Autodesk Inventor part; units mm, degrees
ref_plane "Work Plane1" through (34.6017, 22.9, 27.7) normal (0, 0, 1) x (0, -1, 0)
ref_plane "Work Plane3" through (19.1, 22.9, 27.7) normal (0, -1, 0) x (1, 0, 0)
ref_plane "Work Plane4" through (53.9, 4.4, -9.45) normal (1, 0, 0) x (0, 1, 0)
ref_plane "Work Plane1" through (34.6017, 22.9, 27.7) normal (0, 0, 1) x (0, -1, 0)
sketch "Sketch1" plane through (34.6017, 22.9, 27.7) normal (0, 0, 1) x (0, -1, 0)
  line L0 (-22.65, -5.5017) -> (22.65, -5.5017)
  line L1 (22.65, -5.5017) -> (22.65, -15.5017)
  line L2 (22.65, -15.5017) -> (-22.65, -15.5017)
  line L3 (-22.65, -15.5017) -> (-22.65, -5.5017)
  line L4 (-23.05, -33.7017) -> (-23.05, 15.1916) construction
  line L5 (23.05, 15.1916) -> (23.05, -33.7017) construction
  line L6 (-23.95, -33.6017) -> (-23.95, 15.3983) construction
  line L7 (22.9493, -34.6017) -> (-22.9493, -34.6017) construction
  line L8 (-23.85, -35.5017) -> (23.85, -35.5017) construction
  line L9 (23.05, -33.7017) -> (-23.05, -33.7017) construction
  point P0 (22.9, -34.6017)
  dimension "d0" = 45.3
  dimension "d1" = 10
  dimension "d2" = 0.4
  dimension "d4" = 20
extrude "Extrusion1" add sketch "Sketch1" along normal blind 3
sketch "Sketch2" plane through (19.1, 45.55, 27.7) normal (0, 1, 0) x (1, 0, 0)
  line L0 (10, 0) -> (10, -3)
  line L1 (0, -3) -> (10, -3)
  line L2 (10, -3) -> (10, -0.9)
  line L3 (10, -0.9) -> (0, -0.9)
  line L4 (0, -0.9) -> (0, -3)
  point P0 (-19.1, 27.7)
  dimension "d7" = 2.1
extrude "Extrusion2" add sketch "Sketch2" along normal blind 2
ref_plane "Work Plane3" through (19.1, 22.9, 27.7) normal (0, -1, 0) x (1, 0, 0)
mirror "Mirror2" about plane through (19.1, 22.9, 27.7) normal (0, -1, 0) of "Extrusion2"
sketch "Sketch3" plane through (19.1, 0.25, 27.7) normal (0, -1, 0) x (1, 0, 0)
  line L0 (10, 0.9) -> (0, 0.9)
  line L1 (0, 0) -> (0, 0.9)
  line L2 (10, 0) -> (0, 0)
  line L3 (10, 0) -> (10, 0.9)
  point P0 (-19.1, -27.7)
extrude "Extrusion3" add sketch "Sketch3" along normal blind 0.2
sketch "Sketch4" plane through (19.1, 45.55, 27.7) normal (0, 1, 0) x (1, 0, 0)
  line L0 (0, -0.9) -> (10, -0.9)
  line L1 (10, 0) -> (10, -0.9)
  line L2 (0, 0) -> (10, 0)
  line L3 (0, 0) -> (0, -0.9)
  point P0 (-19.1, 27.7)
extrude "Extrusion4" add sketch "Sketch4" along normal blind 0.2
sketch "Sketch5" plane through (19.1, 47.55, 27.7) normal (0, 1, 0) x (1, 0, 0)
  line L0 (0, -3) -> (10, -3)
  line L1 (10, -3) -> (10, -0.9)
  line L2 (10, -0.9) -> (0, -0.9)
  line L3 (0, -0.9) -> (0, -3)
  point P0 (-19.1, 27.7)
extrude "Extrusion5" add sketch "Sketch5" along normal blind 1.6
sketch "Sketch6" plane through (19.1, -1.75, 30.7) normal (0, -1, 0) x (1, 0, 0)
  line L0 (0, 0) -> (10, 0)
  line L1 (0, -2.1) -> (0, 0)
  line L2 (10, -2.1) -> (0, -2.1)
  line L3 (10, 0) -> (10, -2.1)
  point P0 (-19.1, -30.7)
extrude "Extrusion6" add sketch "Sketch6" along normal blind 1.6
sketch "Sketch7" plane through (29.1, 45.75, 28.6) normal (0, 0, -1) x (-1, 0, 0)
  line L0 (10, 0) -> (10, 3.4)
  line L1 (0, 3.4) -> (10, 3.4)
  line L2 (10, 3.4) -> (10, 1.85)
  line L3 (10, 1.85) -> (0, 1.85)
  line L4 (0, 1.85) -> (0, 3.4)
  point P0 (29.1, -45.75)
  dimension "d20" = 1.55
extrude "Extrusion7" add sketch "Sketch7" along normal up to surface (0.9 mm away)
mirror "Mirror3" about plane through (19.1, 22.9, 27.7) normal (0, -1, 0) of "Extrusion7"
sketch "Sketch8" plane through (19.1, 47.6, 28.6) normal (0, -1, 0) x (1, 0, 0)
  line L0 (0, -0.9) -> (10, -0.9)
  line L1 (10, 0) -> (10, -0.9)
  line L2 (0, 0) -> (10, 0)
  line L3 (0, 0) -> (0, -0.9)
  point P0 (-19.1, -28.6)
extrude "Extrusion8" cut sketch "Sketch8" against normal blind 0.2
sketch "Sketch9" plane through (19.1, -1.8, 27.7) normal (0, 1, 0) x (1, 0, 0)
  line L0 (0, 0) -> (10, 0)
  line L1 (0, -0.9) -> (0, 0)
  line L2 (10, -0.9) -> (0, -0.9)
  line L3 (10, -0.9) -> (10, 0)
  point P0 (-19.1, 27.7)
extrude "Extrusion9" cut sketch "Sketch9" against normal blind 0.2
sketch "Sketch10" plane through (34.6017, 22.9, 30.7) normal (0, 0, 1) x (1, 0, 0)
  line L0 (-5.5017, 26.25) -> (-5.5017, -26.25)
  line L1 (-15.5017, 26.25) -> (-5.5017, 26.25)
  line L2 (-15.5017, -26.25) -> (-15.5017, 26.25)
  line L3 (-5.5017, -26.25) -> (-15.5017, -26.25)
  point P0 (-34.6017, -22.9)
extrude "Extrusion10" add sketch "Sketch10" along normal blind 2
sketch "Sketch11" plane through (29.1, 0.05, 27.7) normal (1, 0, 0) x (0, 0, -1)
  line L0 (0, 45.7) -> (0, 0)
  line L1 (-5, -3.4) -> (-5, 49.1)
  line L2 (-5, 27.85) -> (0, 27.85)
  line L3 (0, 27.85) -> (0, 17.85)
  line L4 (0, 17.85) -> (-5, 17.85)
  line L5 (-5, 17.85) -> (-5, 27.85)
  line L6 (0, 49.1) -> (-5, 49.1)
  point P0 (27.7, -0.05)
  dimension "d29" = 10
  dimension "d37" = 21.25
ref_plane "Work Plane4" through (53.9, 4.4, -9.45) normal (1, 0, 0) x (0, 1, 0)
ref_plane "Work Plane5" through (56.9, 17.9, 20.2) normal (1, 0, 0) x (0, 1, 0)
extrude "Extrusion11" add sketch "Sketch11" along normal up to surface (27.8 mm away)
sketch "Sketch12" plane through (29.1, 17.9, 27.7) normal (0, -1, 0) x (1, 0, 0)
  line L0 (16.8, 0) -> (16.8, 0.8) construction
  line L1 (15.8, 0.8) -> (16.8, 0.8) construction
  line L2 (15, 0) -> (15, 0.8) construction
  line L3 (27.8, 0) -> (27.8, 5) construction
  line L4 (0, 5) -> (27.8, 5) construction
  line L5 (0, 0) -> (0, 5) construction
  line L6 (0, 0) -> (27.8, 0) construction
  line L7 (-34.3067, 0.8) -> (15.8, 0.8) construction
  line L8 (15, 0) -> (15, 0.8) construction
  line L9 (15, 0) -> (15, 0.8)
  line L10 (16.8, 0.8) -> (16.8, 0)
  line L11 (15, 0) -> (16.8, 0)
  line L12 (16.8, 0) -> (16.8, 0.8)
  line L13 (16.8, 0.8) -> (15, 0.8)
  line L14 (15, 0.8) -> (15, 0)
  line L15 (14.9, 0) -> (16.9, 0)
  line L16 (16.9, 0) -> (16.9, 1)
  line L17 (16.9, 1) -> (14.9, 1)
  line L18 (14.9, 1) -> (14.9, 0)
  point P0 (-29.1, -27.7)
  dimension "d32" = 2
  dimension "d33" = 1
  dimension "d34" = 0.1
extrude "Extrusion12" cut sketch "Sketch12" against normal up to next
sketch "Sketch17" plane through (34.6017, 22.9, 32.7) normal (0, 0, 1) x (1, 0, 0)
  circle A0 centre (18.2983, 0) radius 2.15
  point P0 (-34.6017, -22.9)
extrude "Extrusion16" cut sketch "Sketch17" against normal up to next
sketch "Sketch18" plane through (56.9, 17.9, 27.7) normal (1, 0, 0) x (0, 0, -1)
  line L0 (0, 0) -> (-5, 0)
  line L1 (0, 10) -> (0, 0)
  line L2 (-5, 10) -> (0, 10)
  line L3 (-5, 0) -> (-5, 10)
  point P0 (27.7, -17.9)
extrude "Extrusion17" add sketch "Sketch18" along normal blind 3
sketch "Sketch20" plane through (29.1, 17.9, 27.7) normal (0, -1, 0) x (1, 0, 0)
  line L0 (16.9, 0) -> (30.8, 0)
  line L1 (30.8, 5) -> (19.8, 5)
  line L2 (19.8, 5) -> (19.8, 0)
  line L3 (19.8, 0) -> (30.8, 0)
  line L4 (30.8, 0) -> (30.8, 5)
  point P0 (-29.1, -27.7)
  dimension "d51" = 11
extrude "Extrusion18" add sketch "Sketch20" along normal blind 3
sketch "Sketch21" plane through (29.1, 27.9, 32.7) normal (0, 1, 0) x (1, 0, 0)
  line L0 (16.9, 5) -> (30.8, 5)
  line L1 (30.8, 0) -> (19.8, 0)
  line L2 (19.8, 0) -> (19.8, 5)
  line L3 (19.8, 5) -> (30.8, 5)
  line L4 (30.8, 5) -> (30.8, 0)
  point P0 (-29.1, 32.7)
  dimension "d54" = 11
extrude "Extrusion19" add sketch "Sketch21" along normal blind 3
sketch "Sketch22" plane through (34.6017, 22.9, 27.7) normal (0, 0, -1) x (-1, 0, 0)
  line L0 (-14.2983, -8) -> (-22.2983, -8)
  line L1 (-22.2983, -8) -> (-22.2983, -5.5)
  line L2 (-22.2983, -5.5) -> (-14.2983, -5.5)
  line L3 (-14.2983, -5.5) -> (-14.2983, -8)
  point P0 (34.6017, -22.9)
  dimension "d57" = 8
  dimension "d58" = 2.5
extrude "Extrusion20" add sketch "Sketch22" along normal blind 3
sketch "Sketch23" plane through (34.6017, 22.9, 27.7) normal (0, 0, -1) x (-1, 0, 0)
  line L0 (-14.2983, 8) -> (-22.2983, 8)
  line L1 (-22.2983, 8) -> (-22.2983, 5.5)
  line L2 (-22.2983, 5.5) -> (-14.2983, 5.5)
  line L3 (-14.2983, 5.5) -> (-14.2983, 8)
  point P0 (34.6017, -22.9)
  dimension "d61" = 8
  dimension "d62" = 2.5
extrude "Extrusion21" add sketch "Sketch23" along normal blind 3
sketch "Sketch24" plane through (59.9, 17.9, 27.7) normal (1, 0, 0) x (0, 0, -1)
  line L0 (0, 13) -> (0, -3)
  line L1 (-5, 13) -> (0, 13)
  line L2 (-5, -3) -> (-5, 13)
  line L3 (0, -3) -> (-5, -3)
  point P0 (27.7, -17.9)
extrude "Extrusion22" cut sketch "Sketch24" against normal blind 3
sketch "Sketch25" plane through (34.6017, 22.9, 27.7) normal (0, 0, -1) x (-1, 0, 0)
  line L0 (-9.3983, 5) -> (-9.3983, -5)
  line L1 (5.5017, -5) -> (-9.3983, -5)
  line L2 (5.5017, -5) -> (5.5017, -22.85)
  line L3 (15.5017, -22.85) -> (5.5017, -22.85)
  line L4 (15.5017, -22.85) -> (15.5017, 22.85)
  line L5 (5.5017, 22.85) -> (15.5017, 22.85)
  line L6 (5.5017, 22.85) -> (5.5017, 5)
  line L7 (5.5017, 5) -> (-9.3983, 5)
  point P0 (34.6017, -22.9)
extrude "Extrusion23" add sketch "Sketch25" along normal blind 1.3
sketch "Sketch26" plane through (19.1, -3.35, 30.7) normal (0, -1, 0) x (1, 0, 0)
  line L0 (0, -3) -> (0, 2)
  line L1 (10, -3) -> (0, -3)
  line L2 (10, 2) -> (10, -3)
  line L3 (0, 2) -> (10, 2)
  point P0 (-19.1, -30.7)
extrude "Extrusion24" add sketch "Sketch26" along normal blind 1.3
sketch "Sketch27" plane through (19.1, 49.15, 27.7) normal (0, 1, 0) x (1, 0, 0)
  line L0 (10, 0) -> (10, -5)
  line L1 (10, 0) -> (0, 0)
  line L2 (0, -5) -> (0, 0)
  line L3 (10, -5) -> (0, -5)
  point P0 (-19.1, 27.7)
extrude "Extrusion25" add sketch "Sketch27" along normal blind 1.3
sketch "Sketch28" plane through (29.1, 47.8, 27.7) normal (0, 0, -1) x (-1, 0, 0)
  line L0 (0, 0) -> (10, 0)
  line L1 (10, 0) -> (10, 2.65)
  line L2 (0, 2.65) -> (10, 2.65)
  line L3 (0, 0) -> (0, 2.65)
  point P0 (29.1, -47.8)
extrude "Extrusion26" add sketch "Sketch28" along normal blind 1.3
sketch "Sketch29" plane through (29.1, -2, 27.7) normal (0, 0, -1) x (-1, 0, 0)
  line L0 (10, 0) -> (0, 0)
  line L1 (0, 0) -> (0, -2.65)
  line L2 (10, -2.65) -> (0, -2.65)
  line L3 (10, -2.65) -> (10, 0)
  point P0 (29.1, 2)
extrude "Extrusion27" add sketch "Sketch29" along normal blind 1.3
sketch "Sketch30" plane through (34.6017, 22.9, 27.7) normal (0, 0, -1) x (-1, 0, 0)
  circle A0 centre (-18.2983, 0) radius 2.15
  line L0 (-22.2983, 5.5) -> (-22.2983, -5.5)
  line L1 (-22.2983, -5.5) -> (-14.2983, -5.5)
  line L2 (-14.2983, -5) -> (-14.2983, -5.5)
  line L3 (-11.3983, -5) -> (-14.2983, -5)
  line L4 (-11.3983, -5) -> (-11.3983, 5)
  line L5 (-11.3983, 5) -> (-14.2983, 5)
  line L6 (-14.2983, 5) -> (-14.2983, 5.5)
  line L7 (-14.2983, 5.5) -> (-22.2983, 5.5)
  point P0 (34.6017, -22.9)
extrude "Extrusion28" add sketch "Sketch30" along normal blind 1.3
properties part number "LongAxisTopClamp"
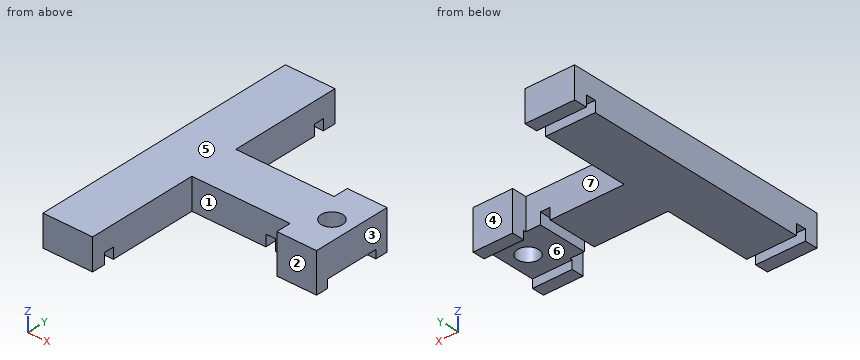
Could you check a few things on this model? Use its own coordinates, in mm. Face numbers are marked on the shaded views. A direction names the side the tool comes from. Coordinates: 2 decimals unless noted, no trailing zeros. Write each loop counter-clockwise with the first axis right and the second up, starting at its lowest first coordinate (ties: lowest second). Pieces come first, ordered by that corner, then holes. Notation, with made-up numbers: (-25.75, 64) -> (-11.75, 64) arc R14 cw to (-11.75, 79) -> close; hole circle Ø9 at (-1.5, 34.5). An arc over 180 degrees is marked (long way). Return JSON: item names as keys, results as strings.
(1) Which directions (+Z, -Z, +X, -X, +Y, -Y) give clear straight access to the entire face, cutting with the end or side of a thin tool? Please do the marked faces 1, 2, 3 and 4.
Numbers:
{"face 1": "+Z, -Z, -Y", "face 2": "+Z, -Z, +X, -Y", "face 3": "+Z, -Z, +X, +Y, -Y", "face 4": "+Z, -Z, +X, +Y"}
(2) We'd pull the mould along Y, two halves only. Please class the marked faces 5, 6 and 7: +Y half, -Y half, draft (parallel to the pull), parting line (faces both ways), or undercut.
Numbers:
{"face 5": "draft", "face 6": "undercut", "face 7": "+Y half"}
(3) Imagine slicing it at B-B, the plane x = 52.9. Please give me the cut outline in (y, z), then the cut area to 3 significant figures.
Numbers:
{"outline": "(14.9, 24.7) -> (17.4, 24.7) -> (17.4, 26.4) -> (20.75, 26.4) -> (20.75, 32.7) -> (14.9, 32.7) -> close; (25.05, 26.4) -> (28.4, 26.4) -> (28.4, 24.7) -> (30.9, 24.7) -> (30.9, 32.7) -> (25.05, 32.7) -> close", "area": "82.2 mm2"}
(4) I need wall thicknesses on L1, parallel to Y at x = 22, z = 28.25; L2, parallel to Y at x = 52.9, z = 29.5; L3, parallel to X at y = 22.9, z = 29. Which ranges of each line are inside material? Lowest first, please.
Numbers:
{"L1": "y = -4.65 to -2, 0.05 to 45.75, 47.8 to 50.45", "L2": "y = 14.9 to 20.75, 25.05 to 30.9", "L3": "x = 19.1 to 50.75, 55.05 to 56.9"}
(5) I'm going to push flat-ended pins straight in: pin 1 (1.6 mm diameter, centred on x = 45.5, y = 21.5, fed in from -Z); pin 2 (1.4 mm diameter, centred on x = 54, z = 25, fed in from +Y); pin 3 (1.4 mm diameter, centred on x = 51.5, z = 25.5, fed in from -Y). Where does each tip first touch, or does it pass through?
Numbers:
{"pin 1": "stops at z = 26.4", "pin 2": "stops at y = 30.9", "pin 3": "stops at y = 14.9"}
(6) Imagine slicing it at A-A, the plane y = 22.9. Please give me the cut outline in (x, z), then the cut area to 3 significant figures.
Numbers:
{"outline": "(19.1, 26.4) -> (44, 26.4) -> (44, 28.7) -> (46, 28.7) -> (46, 26.4) -> (50.75, 26.4) -> (50.75, 32.7) -> (19.1, 32.7) -> close; (55.05, 26.4) -> (56.9, 26.4) -> (56.9, 32.7) -> (55.05, 32.7) -> close", "area": "206 mm2"}
(7) Imagine slicing it at D-D, the plane z = 25.25. Please give me the cut outline in (x, y).
Numbers:
{"outline": "(48.9, 14.9) -> (56.9, 14.9) -> (56.9, 17.4) -> (48.9, 17.4) -> close; (48.9, 28.4) -> (56.9, 28.4) -> (56.9, 30.9) -> (48.9, 30.9) -> close"}
(8) Imagine slicing it at C-C, the plane z = 31.75. Please give me the cut outline in (x, y), then the cut area to 3 significant figures.
Numbers:
{"outline": "(19.1, -4.65) -> (29.1, -4.65) -> (29.1, 17.9) -> (48.9, 17.9) -> (48.9, 14.9) -> (56.9, 14.9) -> (56.9, 30.9) -> (48.9, 30.9) -> (48.9, 27.9) -> (29.1, 27.9) -> (29.1, 50.45) -> (19.1, 50.45) -> close; hole circle Ø4.3 at (52.9, 22.9)", "area": "862 mm2"}
